Part model, mm, in its own coordinate system. A direction names the side the tool comes from. Give positions to 0.01 mm unless a question says otherwise; leave off trailing zeros. Order: outer loops, then holes, each group sorted by start corner. A loop starts at its lowest first (then second) coordinate and runs counter-clockwise, first axis right, second up.
1. Drop flat-ended pins along their axis: pin 1 Ø2 at (x, z) = (0.5, 5) entering from +Y; pin 2 Ø1.5 at (y, z) = (0, -4.5) entering from -X; pin 3 Ø4 at (x, y) = (2.5, -16) entering from -Z. Give the stop position or say it passes through.
2. Slice it at B-B on y = 0. List the corners of the cut face in (x, z), and give its area (3 significant figures).
3. Slice it at C-C on z = -6.5. List the corners of the cut face in (x, y), and give its area (3 significant figures).
4. Slice it at A-A on z = 0. List the corners of the cut face in (x, y).
5. Slice it at D-D on x = -1.75. List the corners of the cut face in (y, z).
6. Probe line 1 (Y direction, x = -0.5, z = 0.5); line 2 (Y direction, x = 0.75, z = 4); line 3 (Y direction, x = 1, z = 15) (3 decimals). List the from-to ranges inside material, lowest first.
7. Which spindle directions (+Z, -Z, +X, -X, +Y, -Y) get a long thin tool onto all of the face, cutting with end or side? Do faces 3 (the flat face through (0, -1.4, 0.3)), 4 (the flat face through (1, -2, 0)). Say none if no direction does.
8. Mould opens along Y. For faces 1 (the flat face through (2, -1.4, 0.3)), 2 (the cylindrical face through (0.056, -23.977, 1.055)) say: +Y half, -Y half, draft (parallel to the pull), parting line (faces both ways), or undercut.
Autodesk Inventor part; units mm, degrees
ref_plane "YZ Plane" through (0, 0, 0) normal (1, 0, 0) x (0, 1, 0)
ref_plane "XZ Plane" through (0, 0, 0) normal (0, 1, 0) x (-1, 0, 0)
ref_plane "XY Plane" through (0, 0, 0) normal (0, 0, 1) x (1, 0, 0)
sketch "Boceto1" plane through (0, 0, 0) normal (1, 0, 0) x (0, 1, 0)
  line L0 (2, 23) -> (-2, 23)
  line L1 (-2, 23) -> (-2, -23)
  line L2 (-2, -23) -> (2, -23)
  line L3 (2, -23) -> (2, 23)
  circle A0 centre (0, 0) radius 1.25
  dimension "d0" = 4
  dimension "d1" = 46
  dimension "d2" = 2
  dimension "d3" = 23
  dimension "d4" = 2.5
extrude "Extrusión1" add sketch "Boceto1" along normal blind 2
sketch "Boceto2" plane through (0, 0, 0) normal (1, 0, 0) x (0, 1, 0)
  circle A0 centre (0, 0) radius 24
  circle A1 centre (0, 0) radius 23
  dimension "d7" = 48
  dimension "d8" = 46
extrude "Extrusión2" add sketch "Boceto2" along normal mid plane 8
properties part number "Molde2" material "Nilón 6/6"
Data:
1. pin 1: stops at y = 23.66
1. pin 2: stops at x = 0
1. pin 3: stops at z = -19.49
2. outline: (-4, -24) - (4, -24) - (4, -23) - (2, -23) - (2, -1.25) - (0, -1.25) - (0, -23) - (-4, -23) - close; (-4, 23) - (0, 23) - (0, 1.25) - (2, 1.25) - (2, 23) - (4, 23) - (4, 24) - (-4, 24) - close
2. area: 103 mm2
3. outline: (-4, -23.1) - (4, -23.1) - (4, -22.06) - (-4, -22.06) - close; (-4, 22.06) - (4, 22.06) - (4, 23.1) - (-4, 23.1) - close; (0, -2) - (2, -2) - (2, 2) - (0, 2) - close
3. area: 24.6 mm2
4. outline: (-4, -24) - (4, -24) - (4, -23) - (-4, -23) - close; (-4, 23) - (4, 23) - (4, 24) - (-4, 24) - close; (0, -2) - (2, -2) - (2, -1.25) - (0, -1.25) - close; (0, 1.25) - (2, 1.25) - (2, 2) - (0, 2) - close
5. outline: circle Ø48 at (0, 0); hole circle Ø46 at (0, 0)
6. line 1: y = -23.99 to -22.99, 22.99 to 23.99
6. line 2: y = -23.66 to -22.65, -2 to 2, 22.65 to 23.66
6. line 3: y = -18.735 to -17.436, -2 to 2, 17.436 to 18.735
7. face 3: -X
7. face 4: +X, -X
8. face 1: undercut
8. face 2: parting line
